Geometry check sheet. Reference: the model listing, model coordinates, mm. A direction names the side the tool comes from. Round coordinates to 2 decimals unless told otherwise and drop trailing zeros. Write each loop counter-clockwise with the first axis right and the second up, starting at its lowest first coordinate (ties: lowest second). Pieces come first, ordered by that corner, then holes. Notation, with made-up numbers: (83, -13) -> (105, -13) arc R5 ccw to (105, -7) -> close; hole circle Ø2 at (-7, -33). An arc over 180 degrees is marked (long way). Use a Markdown table: item, result.
Autodesk Inventor part; units mm, degrees
ref_plane "YZ Plane" through (0, 0, 0) normal (1, 0, 0) x (0, 1, 0)
ref_plane "XZ Plane" through (0, 0, 0) normal (0, 1, 0) x (-1, 0, 0)
ref_plane "XY Plane" through (0, 0, 0) normal (0, 0, 1) x (1, 0, 0)
sketch "Sketch1" plane through (0, 0, 0) normal (0, 1, 0) x (-1, 0, 0)
  circle A0 centre (0, -0.5) radius 5.1
  line L0 (5.0754, 0) -> (13, 0)
  line L1 (13, 0) -> (13, 8)
  line L2 (13, 8) -> (-13, 8)
  line L3 (-13, 8) -> (-13, 0)
  line L4 (-13, 0) -> (-5.0754, 0)
  point P0 (0, 0)
  dimension "d0" = 10.2
  dimension "d1" = 0.5
  dimension "d2" = 26
  dimension "d3" = 13
  dimension "d4" = 8
extrude "Extrusion1" add sketch "Sketch1" along normal blind 20 contours A0 L4 L3 L2 L1 L0
sketch "Sketch2" plane through (-5.0754, 0, 0) normal (0, 0, -1) x (-1, 0, 0)
  line L0 (0, 0) -> (7.9246, 0)
  line L1 (7.9246, 0) -> (7.9246, 20)
  line L2 (-18.0754, 0) -> (-10.1509, 0)
  line L3 (-10.1509, 0) -> (-10.1509, 20)
  line L4 (-18.0754, 20) -> (-10.1509, 20)
  line L5 (-18.0754, 0) -> (-18.0754, 20)
  circle A0 centre (-14.0754, 10) radius 2.25
  circle A1 centre (3.9246, 10) radius 2.25
  point P0 (-5.0754, 0)
  dimension "d8" = 4.5
  dimension "d9" = 18
  dimension "d10" = 4
  dimension "d11" = 10
extrude "Extrusion2" cut sketch "Sketch2" against normal up to surface (8 mm away) contours A0 | A1
sketch "Sketch3" plane through (-13, 0, 8) normal (0, 0, 1) x (1, 0, 0)
  circle A0 centre (4, 10) radius 2.25
  circle A1 centre (22, 10) radius 2.25
  circle A2 centre (4, 10) radius 2.25
  circle A3 centre (4, 10) radius 4
  circle A4 centre (22, 10) radius 4
  point P0 (13, 0)
  dimension "d14" = 8
extrude "Extrusion3" cut sketch "Sketch3" against normal blind 4
properties part number "ZAxisRodClampTop" material "ABS Plastic"
(1) Section check B-B on z = 1.75. Record the cut outline in (x, y).
A:
| item | result |
|---|---|
| outline | (-13, 0) -> (-4.58, 0) -> (-4.58, 20) -> (-13, 20) -> close; (4.58, 0) -> (13, 0) -> (13, 20) -> (4.58, 20) -> close; hole circle Ø4.5 at (-9, 10); hole circle Ø4.5 at (9, 10) |
(2) Section check C-C on y = 15.5. Record the cut outline in (x, z), plus the area to 3 significant figures.
A:
| item | result |
|---|---|
| outline | (-13, 0) -> (-5.08, 0) arc R5.1 cw to (5.08, 0) -> (13, 0) -> (13, 8) -> (-13, 8) -> close |
| area | 172 mm2 |
(3) Thickness scan on line 1 (Y direction, x = -9, z = 5.35); line 2 (X direction, y = 12.5, z = 0.5); line 3 (Y direction, x = -9, z = 2.05). Record the ranges inside material, lowest first.
A:
| item | result |
|---|---|
| line 1 | y = 0 to 6, 14 to 20 |
| line 2 | x = -13 to -5, 5 to 13 |
| line 3 | y = 0 to 7.75, 12.25 to 20 |
(4) Release check for a two-part mould opening along X. For faces 3 (the face through (0, 0, 5)), 4 (the face through (10.66, 11.52, 1.97)), 5 (the face through (-13, 10, 3)) record: +X half, -X half, draft (parallel to the pull), parting line (faces both ways), or undercut.
A:
| item | result |
|---|---|
| face 3 | draft |
| face 4 | undercut |
| face 5 | -X half |
(5) Section check D-D on y = 8.75. Record the cut outline in (x, z).
A:
| item | result |
|---|---|
| outline | (-13, 0) -> (-10.87, 0) -> (-10.87, 4) -> (-12.8, 4) -> (-12.8, 8) -> (-13, 8) -> close; (-7.13, 0) -> (-5.08, 0) arc R5.1 cw to (5.08, 0) -> (7.13, 0) -> (7.13, 4) -> (5.2, 4) -> (5.2, 8) -> (-5.2, 8) -> (-5.2, 4) -> (-7.13, 4) -> close; (10.87, 0) -> (13, 0) -> (13, 8) -> (12.8, 8) -> (12.8, 4) -> (10.87, 4) -> close |
(6) Section check A-A on x = -9. Record the cut outline in (y, z).
A:
| item | result |
|---|---|
| outline | (0, 0) -> (7.75, 0) -> (7.75, 4) -> (6, 4) -> (6, 8) -> (0, 8) -> close; (12.25, 0) -> (20, 0) -> (20, 8) -> (14, 8) -> (14, 4) -> (12.25, 4) -> close |
(7) Gauge pin test, flat ends, axial feed: pin 1 Ø7 at (x, y) = (-9, 10) entering from -Z; pin 2 Ø2.5 at (x, y) = (7.5, 8) entering from +Z; pin 3 Ø6 at (x, y) = (1.5, 16) entering from -Z. Record the tip position at first contact, or that the pin passes through.
A:
| item | result |
|---|---|
| pin 1 | stops at z = 0 |
| pin 2 | stops at z = 4 |
| pin 3 | stops at z = 1.9 |
(8) Access from +Z, -Z, +X, -X, +Y, -Y to the whole of each face (thin tool, end or side, straight path). Record for faces 1 (the face through (0, 20, 5)), 2 (the face through (-7, 8, 4)).
A:
| item | result |
|---|---|
| face 1 | +Z, -Z, +X, -X, +Y |
| face 2 | +Z |
